Can you work these out from the drawing? Everything is in mm from the part's minimum corner. A direction names the side the tool comes from. Give positions to 0.01 mm unless a question says otherwise; leave off trailing zeros. Loops run counter-clockwise (first coordinate to the right, second up) from the corner with the lowest first, then second, coordinate; pieces in that order, holes last. Notation, with made-up numbers: (61.5, -16.5) -> (82.5, -16.5) arc R19 cw to (82.5, 3.5) -> close; hole circle Ø5 at (50.5, -36.5). An arc over 180 degrees is marked (long way). Return JSON: item names as keys, results as strings. Group by question number.
Q1. I need wall thicknesses on line 1 along Y through (x, z) = (116.5, 59.5); line 2 along X through (y, z) = (304, 80); line 3 along X through (y, z) = (324.5, 26). Which ranges of each line are inside material? Lowest first, please. Write a range as [from, to].
Q2. Will these pins go through, and if not, where does the flat tip stop? pin 1 (15.5 mm diameter, centred on x = 174.5, z = 92, fed in from -Y); pin 2 (2 mm diameter, centred on x = 348.5, y = 305, fed in from +Z); pin 3 (4 mm diameter, centred on y = 226, z = 32, fed in from +X).
Q3. Suppose I cut it at D-D, the plane z = 46. Please give me the cut outline in (x, y).
Q4. Which directions (+Z, -Z, +X, -X, +Y, -Y) give clear straight access to the entire face, cutting with the end or side of a thin tool? Please do the marked faces 1, 2, 3 and 4.
Q5. Suppose I cut it at A-A, the plane x = 281. Please give me the cut outline in (y, z).
Q6. Suppose I cut it at B-B, the plane z = 80. Please give me the cut outline in (x, y).
Q7. Thinking about a two-plate mould opening in Y: for the marked faces 5, 6, 7 and 8, which applies, pulls with the +Y half, pulls with the -Y half, needs draft (parallel to the pull), parting line crosses it, or undercut?
Q8. Suppose I cut it at C-C, the plane y = 131. Please give me the cut outline in (x, z), and give its area (3 significant figures).
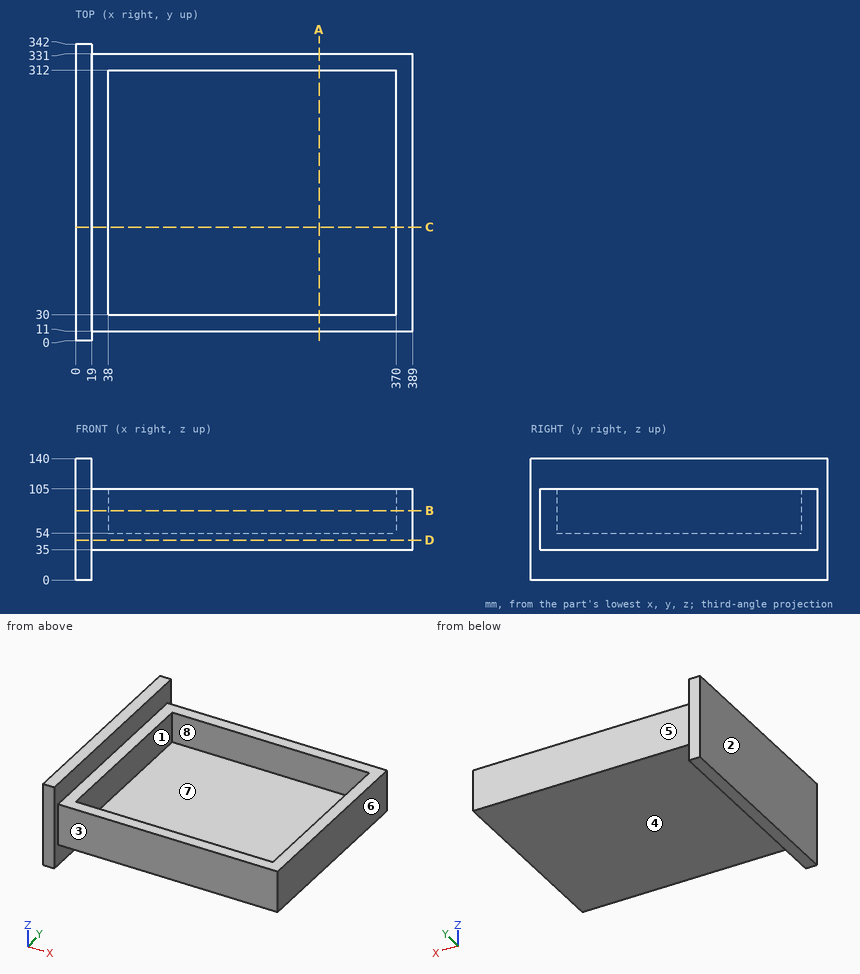
Ans:
{
 "1": {"line 1": "y = [11, 30], [312, 331]", "line 2": "x = [0, 38], [370, 389]", "line 3": "x = [0, 19]"},
 "2": {"pin 1": "stops at y = 11", "pin 2": "stops at z = 54", "pin 3": "stops at x = 19"},
 "3": {"outline": "(0, 0) -> (19, 0) -> (19, 11) -> (389, 11) -> (389, 331) -> (19, 331) -> (19, 342) -> (0, 342) -> close"},
 "4": {"face 1": "+Z", "face 2": "+Z, -Z, -X, +Y, -Y", "face 3": "+Z, -Z, +X, -Y", "face 4": "-Z, +X, +Y, -Y"},
 "5": {"outline": "(11, 35) -> (331, 35) -> (331, 105) -> (312, 105) -> (312, 54) -> (30, 54) -> (30, 105) -> (11, 105) -> close"},
 "6": {"outline": "(0, 0) -> (19, 0) -> (19, 11) -> (389, 11) -> (389, 331) -> (19, 331) -> (19, 342) -> (0, 342) -> close; hole (38, 30) -> (370, 30) -> (370, 312) -> (38, 312) -> close"},
 "7": {"face 5": "pulls with the +Y half", "face 6": "needs draft", "face 7": "undercut", "face 8": "undercut"},
 "8": {"outline": "(0, 0) -> (19, 0) -> (19, 35) -> (389, 35) -> (389, 105) -> (370, 105) -> (370, 54) -> (38, 54) -> (38, 105) -> (19, 105) -> (19, 140) -> (0, 140) -> close", "area": "11,600 mm^2"}
}
